```python
from build123d import *

# Parameters (mm, degrees)
EXTRUDE_1_DEPTH     = 32
EXTRUDE_2_DEPTH     = 30.4
SKETCH_3_W          = 0.8
SKETCH_3_H          = 32
EXTRUDE_3_DEPTH     = 0.6
SKETCH_4_W          = 0.8
SKETCH_4_H          = 32
EXTRUDE_4_DEPTH     = 0.6
SKETCH_5_W          = 11.8
SKETCH_5_H          = 30.4
SKETCH_5_W_2        = 11
EXTRUDE_11_DEPTH    = 0.6
SKETCH_6_R          = 1.6
CUT_EXTRUDE_1_DEPTH = 70.561196079
SKETCH_7_R          = 15
CUT_EXTRUDE_2_DEPTH = 3
SKETCH_8_R          = 3.675878391
CUT_EXTRUDE_3_DEPTH = 10
CUT_EXTRUDE_4_DEPTH = 77.212597384


with BuildPart() as part:
    # 草图1 → 凸台-拉伸1 (new body)
    with BuildSketch(Plane.XY):
        Polygon((-40.6, 33), (-40.6, 0), (-3, 0), (-3, -7), (0, -7), (0, 1.3), (-12, 1.3), (-12, 1.9), (-12.8, 1.9), (-12.8, 1.3), (-23, 1.3), (-23, 1.9), (-23.8, 1.9), (-23.8, 1.3), (-39.6, 1.3), (-39.6, 31.7), (-23.8, 31.7), (-23.8, 30.9), (-23, 30.9), (-23, 31.7), (-12.8, 31.7), (-12.8, 30.9), (-12, 30.9), (-12, 31.7), (0, 31.7), (0, 40), (-3, 40), (-3, 33), (-23, 33), (-23, 48.225966529), (-10.836350524, 48.225966529), (-10.836350524, 49), (-23.8, 49), (-23.8, 33), align=None)
    extrude(amount=EXTRUDE_1_DEPTH)

    # 草图2 → 凸台-拉伸2 (add)
    with BuildSketch(Plane.XZ.offset(-31.7)):
        Polygon((-23.8, 0), (-29.4, 32), (-28.6, 32), (-23, 0), align=None)
    extrude(amount=EXTRUDE_2_DEPTH)

    # 草图3 → 凸台-拉伸3 (add)
    with BuildSketch(Plane.XZ.offset(-31.7)):
        with Locations((-29, 16)):
            Rectangle(SKETCH_3_W, SKETCH_3_H)
    extrude(amount=EXTRUDE_3_DEPTH)

    # 草图4 → 凸台-拉伸4 (add)
    with BuildSketch(Plane(origin=(0, 1.3, 0), x_dir=(1, 0, 0), z_dir=(0, 1, 0))):
        with Locations((-29, -16)):
            Rectangle(SKETCH_4_W, SKETCH_4_H)
    extrude(amount=EXTRUDE_4_DEPTH)

    # 草图5 → 凸台-拉伸11 (add)
    with BuildSketch(Plane(origin=(0, 0, 0), x_dir=(-1, 0, 0), z_dir=(0, 0, -1))):
        with Locations((17.9, 16.5)):
            Rectangle(SKETCH_5_W, SKETCH_5_H)
        with Locations((34.1, 16.5)):
            Rectangle(SKETCH_5_W_2, SKETCH_5_H)
    extrude(amount=-EXTRUDE_11_DEPTH)

    # 草图6 → 切除-拉伸1 (cut, through all)
    with BuildSketch(Plane.ZY.offset(3)):
        with Locations((14.4, 36.855019001)):
            Circle(SKETCH_6_R)
        with Locations(Location((14.4, -3.855019001, 0), (0, 0, 180))):
            Circle(SKETCH_6_R)
    extrude(amount=-CUT_EXTRUDE_1_DEPTH, mode=Mode.SUBTRACT)

    # 草图7 → 切除-拉伸2 (cut)
    with BuildSketch(Plane.ZY.offset(40.6)):
        with Locations((16, 16.5)):
            Circle(SKETCH_7_R)
    extrude(amount=-CUT_EXTRUDE_2_DEPTH, mode=Mode.SUBTRACT)

    # 草图8 → 切除-拉伸3 (cut)
    with BuildSketch(Plane.ZY.offset(23.8)):
        with Locations((14.4, 36.855019001)):
            Circle(SKETCH_8_R)
    extrude(amount=-CUT_EXTRUDE_3_DEPTH, mode=Mode.SUBTRACT)

    # 草图9 → 切除-拉伸4 (cut, through all)
    with BuildSketch(Plane.XZ.offset(7)):
        Polygon((-12.8, 32), (0.069065174, 32), (0.069065174, 30.4), align=None)
    extrude(amount=-CUT_EXTRUDE_4_DEPTH, mode=Mode.SUBTRACT)


solid = part.part
```
Input: part model. Units: mm. Frame: model coordinates. A direction names the side the tool comes from. Give positions to 0.01 mm unless a question says otherwise; leave off trailing zeros. Write each loop counter-clockwise with the first axis right and the second up, starting at its lowest first coordinate (ties: lowest second). Pieces come first, ordered by that corner, then holes. Notation, with made-up numbers: (40, 19) - (79, 19) arc R27 cw to (79, 35) - close; hole circle Ø3 at (63.5, -4). An arc over 180 degrees is marked (long way). Write item = value, one per line. Start each with the question number.
1) Draft query along Y for faces 5 (the face through (-34, 1.3, 16)), 6 (the face through (-40.6, 26, 28)), 7 (the face through (-25, 31.7, 24)). Return one class per face: pulls with the +Y half, pulls with the -Y half, needs draft (parallel to the pull), parting line crosses it, or undercut.
2) Pin query (flat end, axial travel): pin 1 (9.5 mm diameter, centred on x = -18, z = 15, fed in from -Y); pin 2 (1.9 mm diameter, centred on y = -3.86, z = 14.4, fed in from -X); pin 3 (2 mm diameter, centred on y = 43, z = 7.5, fed in from +X); pin 4 (8.5 mm diameter, centred on x = -36, z = 17, fed in from +Y). Return the tip coordinate at first contact, or that it passes through.
3) Material intervals for L1, parallel to Y at x = -20.5, z = 19; L2, parallel to Y at x = -2.3, z = 14.4; L3, parallel to Y at x = -39, z = 16, sorted ascending. Write a range as [from, to].
4) Cut plane B-B (y = 16.5). Return loops of the section in (x, z) (3 decimals).
5) Cut plane C-C (x = -33). Return loops of the section in (y, z).
6) Reachability of faces 1 (the face through (-17, 48.226, 16)), 2 (the face through (-27, 1.3, 7)), 3 (the face through (-25, 1.3, 24)), 4 (the face through (-23.406, 33.267, 13.603)) from +Z, -Z, +X, -X, +Y, -Y: full face, straight path, thin tool, end or side. Return the list, or none.
7) Cut plane D-D (z = 14.4). Give the number of separate pieces and of enclosed holes in the cut face, and give its area (3 significant figures).
8) Cut plane A-A (x = -14.5). Return loops of the section in (y, z).
Answers follow:
q1.face_5 = undercut
q1.face_6 = needs draft
q1.face_7 = undercut
q2.pin_1 = 0
q2.pin_2 = through
q2.pin_3 = -23
q2.pin_4 = 33
q3.L1 = [0, 1.3], [31.7, 33], [48.23, 49]
q3.L2 = [-7, -5.46], [-2.26, 1.3], [31.7, 35.26], [38.46, 40]
q3.L3 = [0, 1.3], [31.7, 33]
q4.outline = (-40.6, 0) - (-28.6, 0) - (-28.6, 0.6) - (-39.6, 0.6) - (-39.6, 1) - (-40.6, 1) - close; (-40.6, 31) - (-39.6, 31) - (-39.6, 32) - (-40.6, 32) - close; (-29.4, 32) - (-23.8, 0) - (-12, 0) - (-12, 0.6) - (-23.105, 0.6) - (-28.6, 32) - close
q5.outline = (0, 0) - (33, 0) - (33, 32) - (31.7, 32) - (31.7, 0.6) - (1.3, 0.6) - (1.3, 32) - (0, 32) - close
q6.face_1 = +Z, -Z, +X
q6.face_2 = -Z
q6.face_3 = +Z
q6.face_4 = -X
q7.separate_pieces = 4
q7.enclosed_holes = 0
q7.area = 173 mm^2
q8.outline = (0, 0) - (33, 0) - (33, 32) - (31.7, 32) - (31.7, 0.6) - (1.3, 0.6) - (1.3, 32) - (0, 32) - close; (48.23, 0) - (49, 0) - (49, 32) - (48.23, 32) - close
